Could you check a few things on this model? Use its own coordinates, in mm. Round coordinates to 2 decimals unless told otherwise and drop trailing zeros. Loops run counter-clockwise (first coordinate to the right, second up) from the corner with the lowest first, then second, coordinate; pieces in that order, holes last. Notation, with made-up numbers: (47.25, 43) -> (82.25, 43) arc R30 ccw to (82.25, 82) -> close; hole circle Ø10 at (1, -18.5). An arc over 180 degrees is marked (long way). Write each question's results on one line, items separated by ' | '.
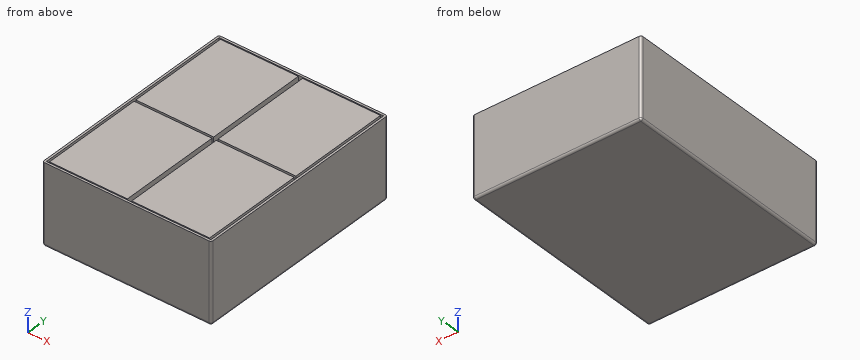
from build123d import *

# Parameters (mm, degrees)
SKETCH_W     = 380
SKETCH_H     = 490
PAD_DEPTH    = 180
THICKNESS_T  = 5
SKETCH001_W  = 180
SKETCH001_H  = 240
PAD001_DEPTH = 180
PAD002_DEPTH = 10


with BuildPart() as part:
    # Sketch → Pad (new body)
    with BuildSketch(Plane.XY):
        Rectangle(SKETCH_W, SKETCH_H)
    extrude(amount=PAD_DEPTH)

    # Thickness
    thickness_openings = [part.faces().sort_by_distance(p)[0] for p in [
        (0, 0, 180),
    ]]
    offset(amount=THICKNESS_T, openings=thickness_openings)

    # Sketch001 (on Face5 of Thickness) → Pad001 (join)
    with BuildSketch(Plane.XY):
        with Locations((-95, 122.5)):
            Rectangle(SKETCH001_W, SKETCH001_H)
        with Locations((95, 122.5)):
            Rectangle(SKETCH001_W, SKETCH001_H)
        with Locations((-95, -122.5)):
            Rectangle(SKETCH001_W, SKETCH001_H)
        with Locations((95, -122.5)):
            Rectangle(SKETCH001_W, SKETCH001_H)
    extrude(amount=PAD001_DEPTH)

    # Sketch001 (on Face5 of Thickness) → Pad002 (join)
    with BuildSketch(Plane.XY):
        with Locations((-95, 122.5)):
            Rectangle(SKETCH001_W, SKETCH001_H)
        with Locations((95, 122.5)):
            Rectangle(SKETCH001_W, SKETCH001_H)
        with Locations((-95, -122.5)):
            Rectangle(SKETCH001_W, SKETCH001_H)
        with Locations((95, -122.5)):
            Rectangle(SKETCH001_W, SKETCH001_H)
    extrude(amount=PAD002_DEPTH)


solid = part.part
1) I need wall thicknesses on line 1 (Y direction, x = -142, z = 32); line 2 (X direction, y = -184, z = 127). Which ranges of each line are inside material? Lowest first, please.
Model answer:
line 1: y = -250 to -245, -242.5 to -2.5, 2.5 to 242.5, 245 to 250 | line 2: x = -195 to -190, -185 to -5, 5 to 185, 190 to 195
2) I want a section at B-B, the plane y = 102. Write out the boundary of the cut face in (x, z), plus the area to 3 significant figures.
Model answer:
outline: (-195, 0) arc R5 ccw to (-190, -5) -> (190, -5) arc R5 ccw to (195, 0) -> (195, 180) -> (190, 180) -> (190, 0) -> (185, 0) -> (185, 180) -> (5, 180) -> (5, 0) -> (-5, 0) -> (-5, 180) -> (-185, 180) -> (-185, 0) -> (-190, 0) -> (-190, 180) -> (-195, 180) -> close | area: 68,500 mm2
3) I want a section at A-A, the plane z = 135.5. Write out the boundary of the cut face in (x, y).
Model answer:
outline: (-195, -245) arc R5 ccw to (-190, -250) -> (190, -250) arc R5 ccw to (195, -245) -> (195, 245) arc R5 ccw to (190, 250) -> (-190, 250) arc R5 ccw to (-195, 245) -> close; (-185, -242.5) -> (-5, -242.5) -> (-5, -2.5) -> (-185, -2.5) -> close; (-185, 2.5) -> (-5, 2.5) -> (-5, 242.5) -> (-185, 242.5) -> close; (5, -242.5) -> (185, -242.5) -> (185, -2.5) -> (5, -2.5) -> close; (5, 2.5) -> (185, 2.5) -> (185, 242.5) -> (5, 242.5) -> close; hole (-190, -245) -> (190, -245) -> (190, 245) -> (-190, 245) -> close
4) I want a section at C-C, the plane x = -74. Write out the boundary of the cut face in (y, z), plus the area to 3 significant figures.
Model answer:
outline: (-250, 0) arc R5 ccw to (-245, -5) -> (245, -5) arc R5 ccw to (250, 0) -> (250, 180) -> (245, 180) -> (245, 0) -> (242.5, 0) -> (242.5, 180) -> (2.5, 180) -> (2.5, 0) -> (-2.5, 0) -> (-2.5, 180) -> (-242.5, 180) -> (-242.5, 0) -> (-245, 0) -> (-245, 180) -> (-250, 180) -> close | area: 90,700 mm2
